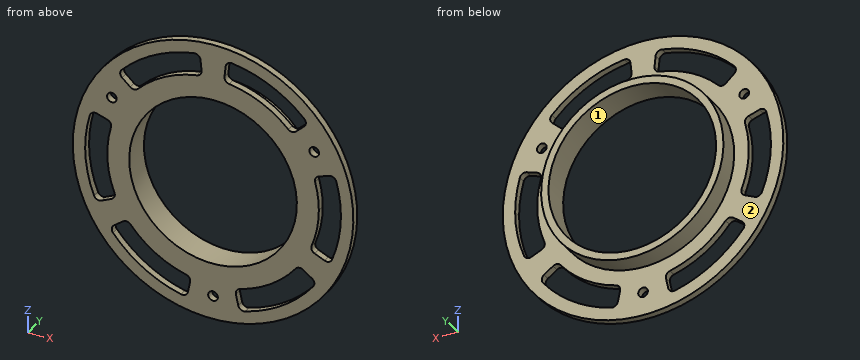
from build123d import *

# Parameters (mm, degrees)
SKETCH1_R               = 76.2
SKETCH1_R_2             = 45.53
BOSS_EXTRUDE1_DEPTH     = 4
CUT_EXTRUDE1_DEPTH      = 108.837284832
CUT_EXTRUDE1_DEPTH_BACK = 108.837284832
SKETCH10_R              = 2.625
CUT_EXTRUDE5_DEPTH      = 6
FILLET1_R               = 3
SKETCH1_12_R            = 49.53
SKETCH1_12_R_2          = 45.53
BOSS_EXTRUDE2_DEPTH     = 15


with BuildPart() as part:
    # Sketch1 → Boss-Extrude1 (new body)
    with BuildSketch(Plane(origin=(0, 0, 0), x_dir=(1, 0, 0), z_dir=(0, 1, 0))):
        with Locations(Location((0, 0, 0), (0, 0, 270))):
            Circle(SKETCH1_R)
        with Locations(Location((0, 0, 0), (0, 0, 270))):
            Circle(SKETCH1_R_2, mode=Mode.SUBTRACT)
    extrude(amount=BOSS_EXTRUDE1_DEPTH)

    # Sketch1_7 → Cut-Extrude1 (cut, two sides: drawn at the far end of the back side and taken through both)
    with BuildSketch(Plane(origin=(0, 0, 0), x_dir=(1, 0, 0), z_dir=(0, 1, 0)).offset(-CUT_EXTRUDE1_DEPTH_BACK)):
        with BuildLine():
            Line((-42.783335499, -38.36795225), (-51.717081111, -46.37970545))
            ThreePointArc((-51.717081111, -46.37970545), (-31.551154407, -61.889079908), (-7.153731292, -69.098174251))
            Line((-7.153731292, -69.098174251), (-5.917976795, -57.16197256))
            ThreePointArc((-5.917976795, -57.16197256), (-26.100924402, -51.198196273), (-42.783335499, -38.36795225))
        make_face()
        with BuildLine():
            Line((-52.462708765, 23.455868036), (-63.417639903, 28.353774095))
            ThreePointArc((-63.417639903, 28.353774095), (-69.373092621, 3.620438719), (-66.024543695, -21.598453327))
            Line((-66.024543695, -21.598453327), (-54.619289089, -17.867479275))
            ThreePointArc((-54.619289089, -17.867479275), (-57.389400801, 2.995034542), (-52.462708765, 23.455868036))
        make_face()
        with BuildLine():
            Line((-11.835953591, 56.235431525), (-14.307462584, 67.978158777))
            ThreePointArc((-14.307462584, 67.978158777), (-37.821938213, 58.268641189), (-56.263908611, 40.744400156))
            Line((-56.263908611, 40.744400156), (-46.544731969, 33.706104523))
            ThreePointArc((-46.544731969, 33.706104523), (-31.288476399, 48.203161731), (-11.835953591, 56.235431525))
        make_face()
        with BuildLine():
            ThreePointArc((56.263908611, 40.744400156), (37.821938213, 58.268641189), (14.307462584, 67.978158777))
            Line((14.307462584, 67.978158777), (11.835953591, 56.235431525))
            ThreePointArc((11.835953591, 56.235431525), (31.288476399, 48.203161731), (46.544731969, 33.706104523))
            Line((46.544731969, 33.706104523), (56.263908611, 40.744400156))
        make_face()
        with BuildLine():
            ThreePointArc((69.4675, 0), (67.938201537, 14.496010767), (63.417639903, 28.353774095))
            Line((63.417639903, 28.353774095), (52.462708765, 23.455868036))
            ThreePointArc((52.462708765, 23.455868036), (56.202376605, 11.991931461), (57.4675, 0))
            ThreePointArc((57.4675, 0), (56.750980397, -9.046534157), (54.619289089, -17.867479275))
            Line((54.619289089, -17.867479275), (66.024543695, -21.598453327))
            ThreePointArc((66.024543695, -21.598453327), (68.601361304, -10.935574222), (69.4675, 0))
        make_face()
        with BuildLine():
            ThreePointArc((7.153731292, -69.098174251), (31.551154407, -61.889079908), (51.717081111, -46.37970545))
            Line((51.717081111, -46.37970545), (42.783335499, -38.36795225))
            ThreePointArc((42.783335499, -38.36795225), (26.100924402, -51.198196273), (5.917976795, -57.16197256))
            Line((5.917976795, -57.16197256), (7.153731292, -69.098174251))
        make_face()
    extrude(amount=CUT_EXTRUDE1_DEPTH + CUT_EXTRUDE1_DEPTH_BACK, mode=Mode.SUBTRACT)

    # Sketch10 → Cut-Extrude5 (cut)
    with BuildSketch(Plane(origin=(0, 4, 0), x_dir=(1, 0, 0), z_dir=(0, 1, 0))):
        with Locations(Location((0, 63.4675, 0), (0, 0, 270))):
            Circle(SKETCH10_R)
        with Locations(Location((54.964467315, -31.73375, 0), (0, 0, 270))):
            Circle(SKETCH10_R)
        with Locations(Location((-54.964467315, -31.73375, 0), (0, 0, 270))):
            Circle(SKETCH10_R)
    extrude(amount=-CUT_EXTRUDE5_DEPTH, mode=Mode.SUBTRACT)

    # Fillet1
    fillet1_edges = [part.edges().sort_by_distance(p)[0] for p in [
        (42.783335499, 2, 38.36795225),
        (5.917976795, 2, 57.16197256),
        (7.153731292, 2, 69.098174251),
        (51.717081111, 2, 46.37970545),
        (52.462708765, 2, -23.455868036),
        (54.619289089, 2, 17.867479275),
        (66.024543695, 2, 21.598453327),
        (63.417639903, 2, -28.353774095),
        (11.835953591, 2, -56.235431525),
        (46.544731969, 2, -33.706104523),
        (56.263908611, 2, -40.744400156),
        (14.307462584, 2, -67.978158777),
        (-46.544731969, 2, -33.706104523),
        (-11.835953591, 2, -56.235431525),
        (-14.307462584, 2, -67.978158777),
        (-56.263908611, 2, -40.744400156),
        (-54.619289089, 2, 17.867479275),
        (-52.462708765, 2, -23.455868036),
        (-63.417639903, 2, -28.353774095),
        (-66.024543695, 2, 21.598453327),
        (-5.917976795, 2, 57.16197256),
        (-42.783335499, 2, 38.36795225),
        (-51.717081111, 2, 46.37970545),
        (-7.153731292, 2, 69.098174251),
    ]]
    fillet(fillet1_edges, radius=FILLET1_R)

    # Sketch1_12 → Boss-Extrude2 (add)
    with BuildSketch(Plane(origin=(0, 0, 0), x_dir=(1, 0, 0), z_dir=(0, 1, 0))):
        with Locations(Location((0, 0, 0), (0, 0, 270))):
            Circle(SKETCH1_12_R)
        with Locations(Location((0, 0, 0), (0, 0, 270))):
            Circle(SKETCH1_12_R_2, mode=Mode.SUBTRACT)
    extrude(amount=BOSS_EXTRUDE2_DEPTH)


solid = part.part
Read the model definition and answer for the solid it produces. Units are mm, in the model's axes. Face numbers are marked on the shaded views. Round coordinates to 2 decimals unless told otherwise and drop trailing zeros. Write each loop counter-clockwise with the first axis right and the second up, starting at its lowest first coordinate (ties: lowest second). Pieces come first, ordered by that corner, then holes. Notation, with made-up numbers: (32.25, 40) - (68.25, 40) arc R15 ccw to (68.25, 45) - close; hole circle Ø1 at (9.5, 9). An arc over 180 degrees is marked (long way). Use a Markdown table: item, result.
(1) Straight lines are drawn through the part: line 1 along X through (y, z) = (10, 0); line 2 along X through (y, z) = (2.5, -25.5); line 3 along X through (y, z) = (1.75, 11). For each, find the intervals that lie inside material, in ascending order. Write a range as [from, to].
Reported:
| item | result |
|---|---|
| line 1 | [-49.53, -45.53], [45.53, 49.53] |
| line 2 | [-71.81, -64.62], [-57.03, -37.72], [37.72, 57.03], [64.62, 71.81] |
| line 3 | [-75.4, -68.59], [-56.4, -44.18], [44.18, 56.4], [68.59, 75.4] |
(2) The mould has two halves that part along X. Classify the marked faces 1 and 2: released by +X, released by -X, zero draft, split by the parting line, or undercut.
Reported:
| item | result |
|---|---|
| face 1 | undercut |
| face 2 | zero draft |
(3) The part is cut by section A-A (x = 0). Write down the section's boundary in (y, z).
Reported:
| item | result |
|---|---|
| outline | (0, -76.2) - (4, -76.2) - (4, -66.09) - (0, -66.09) - close; (0, -60.84) - (4, -60.84) - (4, -49.53) - (15, -49.53) - (15, -45.53) - (0, -45.53) - close; (0, 45.53) - (15, 45.53) - (15, 49.53) - (4, 49.53) - (4, 76.2) - (0, 76.2) - close |
(4) Each of these flat-tipped pins is pushed along its axis until it touches: pin 1 Ø4 at (x, z) = (0, -63.47) entering from +Y; pin 2 Ø8.5 at (x, z) = (54.96, 31.73) entering from +Y; pin 3 Ø2 at (y, z) = (3.5, -37.5) entering from -X; pin 4 Ø8 at (y, z) = (3, 18) entering from -X. Where does it stop, or does it pass through?
Reported:
| item | result |
|---|---|
| pin 1 | through |
| pin 2 | y = 4 |
| pin 3 | x = -66.89 |
| pin 4 | x = -74.9 |
(5) The part is cut by section B-B (z = -18). Write down the section's boundary in (x, y).
Reported:
| item | result |
|---|---|
| outline | (-74.04, 0) - (-67.09, 0) - (-67.09, 4) - (-74.04, 4) - close; (-54.58, 0) - (-41.82, 0) - (-41.82, 15) - (-46.14, 15) - (-46.14, 4) - (-54.58, 4) - close; (41.82, 0) - (54.58, 0) - (54.58, 4) - (46.14, 4) - (46.14, 15) - (41.82, 15) - close; (67.09, 0) - (74.04, 0) - (74.04, 4) - (67.09, 4) - close |
(6) The part is cut by section C-C (y = 11). Write down the section's boundary in (x, z), then the cut area to 3 significant figures.
Reported:
| item | result |
|---|---|
| outline | circle Ø99.06 at (0, 0); hole circle Ø91.06 at (0, 0) |
| area | 1,190 mm2 |
